Work out the finished part from the listing and answer in its coordinate system (mm). Face numbers are marked on the shaded views. A direction names the side the tool comes from. Coordinates: 2 decimals unless noted, no trailing zeros. Write each loop counter-clockwise with the first axis right and the second up, starting at its lowest first coordinate (ties: lowest second). Pieces come first, ordered by that corner, then holes. Notation, with made-up numbers: M 85.25,28 L 94.25,28 A25 cw 94.25,41 Z; hole C 1.5,80.25 d9. An arc over 180 degrees is marked long. Answer as CSV lines item,"result". Start each with the question number.
(1) Find the intervals of material crossed by L1, parallel to Z at x = -17, y = -3; L2, parallel to X at y = 16, z = 11; L3, parallel to X at y = -2, z = 4.5, in increasing order. Write a range as [from, to].
(2) A cutting plane is placed at B-B on y = -9. Give the vertices of the cut face in (x, z) (3 decimals).
(3) The mould has two halves that part along X. Classify the marked faces 5, 6, 7 and 8: released by +X, released by -X, zero draft, split by the parting line, or undercut.
(4) Flat-ended cylindrical pins translate along their axes: P1, Ø7.5, axis at y = 25.5, z = 8, coming from the -X side; P2, Ø1.5, axis at x = -57, z = 13.5, coming from the +Y side; P3, Ø16.5, axis at y = 34.5, z = 5, coming from the +X side; P4, Ø2, axis at x = 17, y = -27, coming from the +Z side. Find the tip coordinate at first contact, or state that the pin passes through.
(5) A cutting plane is placed at D-D on y = 16. Give the vertices of the cut face in (x, z), then the cut area to 3 significant figures.
(6) A cutting plane is placed at A-A on x = -19. Give the vertices of the cut face in (y, z), then the cut area to 3 significant figures.
(7) A cutting plane is placed at C-C on z = 7.5. Give the vertices of the cut face in (x, y), then the cut area to 3 significant figures.
(8) For the marked faces 1, 2, 3 and 4, determine the directions among +Z, -Z, +X, -X, +Y, -Y from which every point of the face is accessible in a straight line to the end or side of a thin tool.
from build123d import *

# Parameters (mm, degrees)
BOSS_EXTRUDE1_DEPTH     = 15
SKETCH2_W               = 24
SKETCH2_H               = 12
BOSS_EXTRUDE2_DEPTH     = 36
SKETCH3_W               = 42
SKETCH3_H               = 18
BOSS_EXTRUDE3_DEPTH     = 15
SKETCH4_R               = 3
CUT_EXTRUDE1_DEPTH      = 34
BOSS_EXTRUDE5_DEPTH     = 18
SKETCH7_R               = 9
BOSS_EXTRUDE8_DEPTH     = 15
CUT_EXTRUDE2_DEPTH      = 90.487429285
CUT_EXTRUDE2_DEPTH_BACK = 90.487429285
SKETCH8_R               = 4.5
FILLET1_R               = 18
FILLET2_R               = 32


with BuildPart() as part:
    # Sketch1 → Boss-Extrude1 (new body)
    with BuildSketch(Plane.XY):
        with BuildLine():
            Line((0, 0), (12, 0))
            Line((12, 0), (12, 40))
            Line((12, 40), (26, 40))
            Line((26, 40), (26, 24.94427191))
            ThreePointArc((26, 24.94427191), (27, 7), (28, 24.94427191))
            Line((28, 24.94427191), (28, 40))
            Line((28, 40), (42, 40))
            Line((42, 40), (42, -36))
            Line((42, -36), (0, -36))
            Line((0, -36), (0, 0))
        make_face()
    extrude(amount=BOSS_EXTRUDE1_DEPTH)

    # Sketch2 → Boss-Extrude2 (add)
    with BuildSketch(Plane(origin=(0, 0, 0), x_dir=(1, 0, 0), z_dir=(0, 1, 0))):
        Polygon((-36, -18), (0, -18), (0, -15), (0, 0), (0, 6), (-36, 6), align=None)
        with Locations((-18, -6)):
            Rectangle(SKETCH2_W, SKETCH2_H, mode=Mode.SUBTRACT)
    extrude(amount=-BOSS_EXTRUDE2_DEPTH)

    # Sketch3 → Boss-Extrude3 (add)
    with BuildSketch(Plane.XY.offset(18)):
        with Locations((-57, -27)):
            Rectangle(SKETCH3_W, SKETCH3_H)
    extrude(amount=-BOSS_EXTRUDE3_DEPTH)

    # Sketch4 → Cut-Extrude1 (cut)
    with BuildSketch(Plane(origin=(42, 0, 0), x_dir=(0, 0, -1), z_dir=(1, 0, 0))):
        with Locations((-7.5, 34)):
            Circle(SKETCH4_R)
    extrude(amount=-CUT_EXTRUDE1_DEPTH, mode=Mode.SUBTRACT)

    # Sketch6 → Boss-Extrude5 (add)
    with BuildSketch(Plane.ZY.offset(78)):
        Polygon((3, -18), (-15, -2), (-15, 10), (0, 10), (0, 1), (18, -15), (18, -18), align=None)
    extrude(amount=-BOSS_EXTRUDE5_DEPTH)

    # Sketch7 → Boss-Extrude8 (add)
    with BuildSketch(Plane.XY):
        with Locations((-69, 10)):
            Circle(SKETCH7_R)
    extrude(amount=-BOSS_EXTRUDE8_DEPTH)

    # Sketch8 → Cut-Extrude2 (cut, two sides: drawn at the far end of the back side and taken through both)
    with BuildSketch(Plane.XY.offset(-CUT_EXTRUDE2_DEPTH_BACK)):
        with Locations((-69.000940425, 9.869897064)):
            Circle(SKETCH8_R)
    extrude(amount=CUT_EXTRUDE2_DEPTH + CUT_EXTRUDE2_DEPTH_BACK, mode=Mode.SUBTRACT)

    # Fillet1
    fillet1_edges = [part.edges().sort_by_distance(p)[0] for p in [
        (-78, -36, 10.5),
    ]]
    fillet(fillet1_edges, radius=FILLET1_R)

    # Fillet2
    fillet2_edges = [part.edges().sort_by_distance(p)[0] for p in [
        (42, -36, 7.5),
    ]]
    fillet(fillet2_edges, radius=FILLET2_R)


solid = part.part
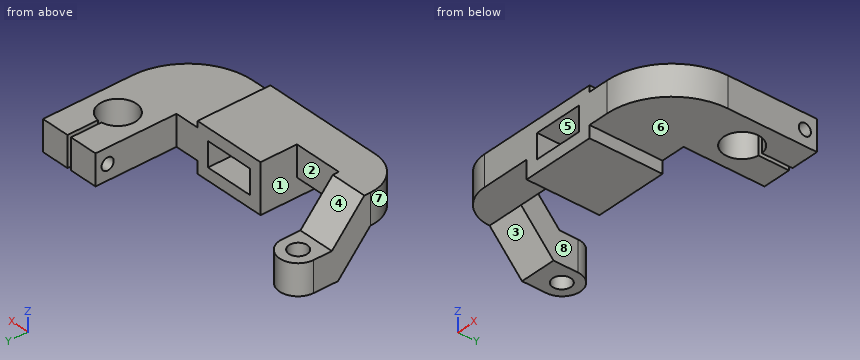
Here are the results:
1,L1,"z = [-6, 0], [12, 18]"
1,L2,"x = [12, 18], [36, 42]"
1,L3,"x = [-36, -30], [-6, 42]"
2,outline,"M -78,-7.125 L -60,-7.125 L -60,11.25 L -78,11.25 Z; M -36,-6 L 0,-6 L 0,0 L 41.607,0 L 41.607,15 L 0,15 L 0,18 L -36,18 Z; hole M -30,0 L -6,0 L -6,12 L -30,12 Z"
3,face 5,"undercut"
3,face 6,"zero draft"
3,face 7,"released by -X"
3,face 8,"undercut"
4,P1,"stops at x = 12"
4,P2,"stops at y = -18"
4,P3,"stops at x = 42"
4,P4,"stops at z = 15"
5,outline,"M -75.71,-15 L -62.29,-15 L -62.29,0 L -75.71,0 Z; M 12,0 L 18,0 L 18,15 L 12,15 Z; M 36,0 L 42,0 L 42,15 L 36,15 Z"
5,area,"381 mm^2"
6,outline,"M -36,-6 L 0,-6 L 0,0 L -36,0 Z; M -36,12 L 0,12 L 0,18 L -36,18 Z"
6,area,"432 mm^2"
7,outline,"M -78,-18 A18 ccw -60,-36 L -30,-36 L -30,0 L -36,0 L -36,-18 L -60,-18 L -60,-5.67 L -78,-5.67 Z; M -6,-36 L 10,-36 A32 ccw 42,-4 L 42,31 L 28,31 L 28,24.94 A9 cw long 26,24.94 L 26,31 L 12,31 L 12,0 L -6,0 Z; M 12,37 L 26,37 L 26,40 L 12,40 Z; M 28,37 L 42,37 L 42,40 L 28,40 Z"
7,area,"3,380 mm^2"
8,face 1,"-Z, +Y"
8,face 2,"+Z, -Z, +Y"
8,face 3,"-Z, -X, -Y"
8,face 4,"+Z, -X, +Y"
